For this review, take the finished solid that the model builds, in its own axes (mm). A direction names the side the tool comes from. Coordinates: 2 decimals unless noted, no trailing zeros.
1) To check wall thickness, follow line 1 along X through (y, z) = (576.5, 35.5); line 2 along Z through (x, y) = (738, 494); line 3 along Z through (x, y) = (744, 565). State the ranges of each line that lie inside material, in increasing order.
2) Insertion check: P1, Ø4, axis at x = 737, y = 604.5, coming from the -Z side; P2, Ø11.5, axis at x = 744.89, y = 575.4, coming from the +Z side; P3, Ø10.5, axis at x = 772.89, y = 575.4, coming from the +Z side. Each pin has a flat end and moves straight along its axis. Give the tip position at first contact, or say it passes through.
3) For faces 1 (the face through (758.96, 594.71, 31.8)), 2 (the face through (750, 473.395, 42)), list the 3-axis set-ups (+Z, -Z, +X, -X, +Y, -Y) from which the entire face can be reached by the end or side of a thin tool; tool diameter is ignored.
4) Mouldability with a two-part tool opening along Y and no side actions: class faces 3 (the face through (786.334, 599.345, 31.58)), 4 (the face through (745, 579.395, 35)) as pulls with the +Y half, pulls with the -Y half, needs draft (parallel to the pull), parting line crosses it, or undercut.
from build123d import *

# Parameters (mm, degrees)
BOSS_EXTRUDE1_DEPTH     = 92
CUT_EXTRUDE1_DEPTH      = 79
CUT_EXTRUDE1_DEPTH_BACK = 118
SKETCH3_OUTSIDE_W       = 130.624
SKETCH3_OUTSIDE_H       = 186.018
CUT_EXTRUDE2_DEPTH      = 81


with BuildPart() as part:
    # Sketch2 → Boss-Extrude1 (new body)
    with BuildSketch(Plane.XY):
        with BuildLine():
            Line((733.88097227, 512.409540482), (733.714590272, 485.398634247))
            ThreePointArc((733.714590272, 485.398634247), (736.969847934, 477.167503112), (744.977198909, 473.39516265))
            Line((744.977198909, 473.39516265), (754.180697278, 473.39516265))
            ThreePointArc((754.180697278, 473.39516265), (754.93321765, 473.712680398), (755.230833309, 474.473291567))
            Line((755.230833309, 474.473291567), (753.644223799, 534.77684994))
            ThreePointArc((753.644223799, 534.77684994), (755.079973826, 538.669205509), (758.892348589, 540.305545534))
            ThreePointArc((758.892348589, 540.305545534), (762.704723352, 538.669205509), (764.140473379, 534.77684994))
            Line((764.140473379, 534.77684994), (762.553863869, 474.473291567))
            ThreePointArc((762.553863869, 474.473291567), (762.851479527, 473.712680398), (763.6039999, 473.39516265))
            Line((763.6039999, 473.39516265), (772.807498269, 473.39516265))
            ThreePointArc((772.807498269, 473.39516265), (780.815918514, 477.166499838), (784.070106906, 485.398634247))
            Line((784.070106906, 485.398634247), (783.903724908, 512.409540482))
            Line((783.903724908, 512.409540482), (783.587761623, 563.703879936))
            ThreePointArc((783.587761623, 563.703879936), (783.77247461, 571.386020865), (784.420563352, 579.043003895))
            Line((784.420563352, 579.043003895), (788.264414586, 619.838080174))
            ThreePointArc((788.264414586, 619.838080174), (788.129918742, 620.240910995), (787.741481052, 620.412602475))
            Line((787.741481052, 620.412602475), (763.947048131, 620.430206642))
            Line((763.947048131, 620.430206642), (762.720599723, 620.430206642))
            ThreePointArc((762.720599723, 620.430206642), (762.341943379, 620.26897154), (762.195758152, 619.884254418))
            Line((762.195758152, 619.884254418), (762.351012345, 598.173946788))
            ThreePointArc((762.351012345, 598.173946788), (758.884364195, 594.707298638), (755.417716045, 598.173946788))
            Line((755.417716045, 598.173946788), (755.572970238, 619.86665025))
            ThreePointArc((755.572970238, 619.86665025), (755.426785011, 620.251367372), (755.048128667, 620.412602475))
            Line((755.048128667, 620.412602475), (753.837649047, 620.412602475))
            Line((753.837649047, 620.412602475), (730.043216126, 620.412602475))
            ThreePointArc((730.043216126, 620.412602475), (729.654778436, 620.240910995), (729.520282592, 619.838080174))
            Line((729.520282592, 619.838080174), (733.364133826, 579.043003895))
            ThreePointArc((733.364133826, 579.043003895), (733.483379901, 577.967121369), (733.593469282, 576.890263363))
            ThreePointArc((733.593469282, 576.890263363), (734.066308334, 570.3049022), (734.196935555, 563.703879936))
            Line((734.196935555, 563.703879936), (733.88097227, 512.409540482))
        make_face()
    extrude(amount=BOSS_EXTRUDE1_DEPTH)

    # Sketch3 outside → Cut-Extrude1 (cut, two sides: drawn at the far end of the back side and taken through both)
    with BuildSketch(Plane(origin=(730.696902853, -4.500952665, 0), x_dir=(0, 0, 1), z_dir=(-0.9999810289222565, 0.006159691192376741, 0)).offset(-CUT_EXTRUDE1_DEPTH_BACK)):
        with Locations((46, 551.577)):
            Rectangle(SKETCH3_OUTSIDE_W, SKETCH3_OUTSIDE_H)
        with BuildLine():
            Line((43.143604537, 477.975011324), (40.424473775, 477.975011324))
            ThreePointArc((40.424473775, 477.975011324), (39.281332513, 493.147025466), (39.432951406, 508.361288404))
            Line((39.432951406, 508.361288404), (40.812056524, 534.581043725))
            ThreePointArc((40.812056524, 534.581043725), (40.67113948, 544.675291647), (39.192711885, 554.661679912))
            ThreePointArc((39.192711885, 554.661679912), (35.60695145, 571.936620339), (32.326521857, 589.272133783))
            ThreePointArc((32.326521857, 589.272133783), (29.707708403, 607.06664821), (28.235119991, 624.992451149))
            Line((28.235119991, 624.992451149), (30.938516025, 624.992451149))
            ThreePointArc((30.938516025, 624.992451149), (34.470259418, 592.692390498), (41.750655625, 561.025957788))
            ThreePointArc((41.750655625, 561.025957788), (44.799963896, 543.735773309), (44.004202882, 526.196801712))
            ThreePointArc((44.004202882, 526.196801712), (41.914294104, 502.115525022), (43.143604537, 477.975011324))
        make_face(mode=Mode.SUBTRACT)
    extrude(amount=CUT_EXTRUDE1_DEPTH + CUT_EXTRUDE1_DEPTH_BACK, mode=Mode.SUBTRACT)

    # Sketch4 → Cut-Extrude2 (cut)
    with BuildSketch(Plane.XY):
        with BuildLine():
            Line((770.830795776, 579.39516265), (774.953901402, 579.39516265))
            ThreePointArc((774.953901402, 579.39516265), (772.892348589, 570.89516265), (770.830795776, 579.39516265))
        make_face()
        with BuildLine():
            Line((742.830795776, 579.39516265), (746.953901402, 579.39516265))
            ThreePointArc((746.953901402, 579.39516265), (744.892348589, 570.89516265), (742.830795776, 579.39516265))
        make_face()
    extrude(amount=CUT_EXTRUDE2_DEPTH, mode=Mode.SUBTRACT)


solid = part.part
Result:
1. line 1: x = 733.63 to 740.53, 749.25 to 768.53, 777.25 to 784.15
1. line 2: z = 39.19 to 41.89
1. line 3: z = 36.08 to 39.4
2. P1: stops at z = 29.28
2. P2: stops at z = 38.24
2. P3: stops at z = 38.08
3. face 1: +Z, -Z
3. face 2: +Z, -Z, +X, -X, -Y
4. face 3: pulls with the -Y half
4. face 4: undercut
